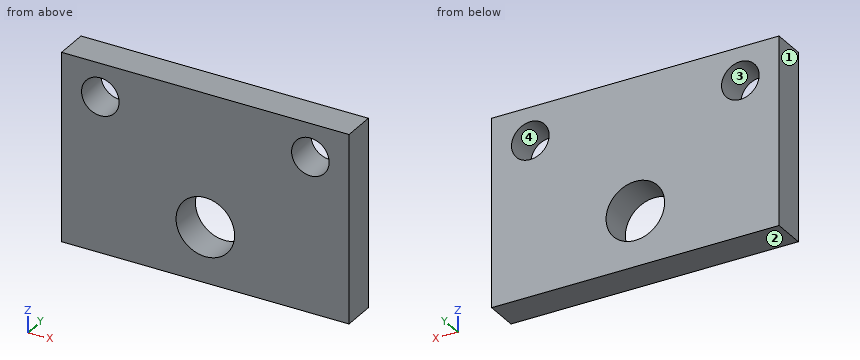
```python
from build123d import *

# Parameters (mm, degrees)
ESBO_O1_W                = 26
ESBO_O1_H                = 17
ESBO_O1_R                = 2.65
RESSALTO_EXTRUS_O1_DEPTH = 3
ESBO_O2_R                = 1.7
CORTE_EXTRUS_O1_DEPTH    = 10


with BuildPart() as part:
    # Esboço1 → Ressalto-extrusão1 (new body)
    with BuildSketch(Plane(origin=(0, 0, 0), x_dir=(1, 0, 0), z_dir=(0, 1, 0))):
        with Locations((13, 8.5)):
            Rectangle(ESBO_O1_W, ESBO_O1_H)
        with Locations((13, 12)):
            Circle(ESBO_O1_R, mode=Mode.SUBTRACT)
    extrude(amount=RESSALTO_EXTRUS_O1_DEPTH)

    # Esboço2 → Corte-extrusão1 (cut)
    with BuildSketch(Plane(origin=(0, 3, 0), x_dir=(1, 0, 0), z_dir=(0, 1, 0))):
        with Locations((3.5, 3)):
            Circle(ESBO_O2_R)
        with Locations((22.5, 3)):
            Circle(ESBO_O2_R)
    extrude(amount=-CORTE_EXTRUS_O1_DEPTH, mode=Mode.SUBTRACT)


solid = part.part
```
The listing builds one solid part. Answer for the finished solid, in the listing's coordinates (mm). Face numbers are marked on the shaded views. Coordinates: 2 decimals unless noted, no trailing zeros. Loops run counter-clockwise (first coordinate to the right, second up) from the corner with the lowest first, then second, coordinate; pieces in that order, holes last. Notation, with made-up numbers: (34.5, -35) -> (48.5, -35) arc R24 cw to (48.5, 4) -> close; hole circle Ø10 at (-6, 65.25). An arc over 180 degrees is marked (long way). Use one line per item in the form item = value. Start each with the question number.
Item 1: The mould has two halves that part along X. Classify the marked faces 1, 2, 3 and 4: released by +X, released by -X, zero draft, split by the parting line, or undercut.
Item 2: The part is cut by section C-C on z = -3. Determine the outline of the cut face in (x, y), then the cut area to 3 significant figures.
Item 3: The part is cut by section A-A on x = 3.5. Determine the outline of the cut face in (y, z), then the cut area to 3 significant figures.
Item 4: The part is cut by section B-B on z = -12. Determine the outline of the cut face in (x, y).
Item 5: Consider L1, parallel to X at y = 1.3, z = -3; L2, parallel to X at y = 1.7, z = -12; L3, parallel to Z at x = 22.5, y = 1. Determine where each line is inside the solid, lowest interval first. Write a range as [from, to].
Item 6: A flat-ended cylindrical pin translates along its axis: pin 1 Ø3 at (x, z) = (13, -12) entering from -Y. Find the tip coordinate at first contact, or state that the pin passes through.
Item 7: The part is cut by section D-D on y = 2.1. Determine the outline of the cut face in (x, z).
Answer key:
q1.face_1 = released by -X
q1.face_2 = zero draft
q1.face_3 = undercut
q1.face_4 = undercut
q2.outline = (0, 0) -> (1.8, 0) -> (1.8, 3) -> (0, 3) -> close; (5.2, 0) -> (20.8, 0) -> (20.8, 3) -> (5.2, 3) -> close; (24.2, 0) -> (26, 0) -> (26, 3) -> (24.2, 3) -> close
q2.area = 57.6 mm2
q3.outline = (0, -17) -> (3, -17) -> (3, -4.7) -> (0, -4.7) -> close; (0, -1.3) -> (3, -1.3) -> (3, 0) -> (0, 0) -> close
q3.area = 40.8 mm2
q4.outline = (0, 0) -> (10.35, 0) -> (10.35, 3) -> (0, 3) -> close; (15.65, 0) -> (26, 0) -> (26, 3) -> (15.65, 3) -> close
q5.L1 = [0, 1.8], [5.2, 20.8], [24.2, 26]
q5.L2 = [0, 10.35], [15.65, 26]
q5.L3 = [-17, -4.7], [-1.3, 0]
q6.pin_1 = through
q7.outline = (0, -17) -> (26, -17) -> (26, 0) -> (0, 0) -> close; hole circle Ø3.4 at (3.5, -3); hole circle Ø5.3 at (13, -12); hole circle Ø3.4 at (22.5, -3)
